Can you work these out from the model? Positions are in its coordinate system, mm. A direction names the side the tool comes from. Give positions to 0.01 mm unless a question says otherwise; leave off trailing zeros. Loops run counter-clockwise (first coordinate to the right, second up) from the corner with the lowest first, then second, coordinate; pieces in that order, holes last. Notation, with made-up numbers: (87.5, 87) -> (91.5, 87) arc R14 ccw to (91.5, 103) -> close; hole circle Ø8 at (-39, -35.75). An arc over 180 degrees is marked (long way). One line per question, with ' | ' between items.
from build123d import *

# Parameters (mm, degrees)
F0_R     = 85
F5_R     = 11
F6_DEPTH = 25
F7_R     = 142.5
F7_R_2   = 11
F7_R_3   = 85
F8_DEPTH = 25


with BuildPart() as f4:
    # F4: sweep along a path in F4_path
    with BuildLine(Plane(origin=(0, 0, 0), x_dir=(0, 1, 0), z_dir=(0, 0, 1))) as f4_path:
        Line((0, 0), (0, -30))
        ThreePointArc((0, -30), (-49.7918471983, -150.2081528017), (-170, -200))
        Line((-170, -200), (-1710, -200))
    # F0 (on Right) → F4 (sweep)
    with BuildSketch(Plane.YZ):
        Circle(F0_R)
    sweep(path=f4_path.line)

    # F5 (on face) → F6 (join)
    with BuildSketch(Plane.XZ.offset(1710)):
        with BuildLine():
            ThreePointArc((84.4, 10.0816665289), (78.6809157211, 32.1607447254), (67.296875, 51.9242777055))
            ThreePointArc((67.296875, 51.9242777055), (57.5, 0), (67.296875, -51.9242777055))
            ThreePointArc((67.296875, -51.9242777055), (78.6809157211, -32.1607447254), (84.4, -10.0816665289))
            ThreePointArc((84.4, -10.0816665289), (69, 0), (84.4, 10.0816665289))
        make_face()
        with BuildLine():
            ThreePointArc((67.296875, -51.9242777055), (226.4202071103, -140.0293635501), (342.5, 0))
            ThreePointArc((342.5, 0), (226.4202071103, 140.0293635501), (67.296875, 51.9242777055))
            ThreePointArc((67.296875, 51.9242777055), (78.6809157211, 32.1607447254), (84.4, 10.0816665289))
            ThreePointArc((84.4, 10.0816665289), (89.2032602919, 6.0249481326), (91, 0))
            ThreePointArc((91, 0), (89.2032602919, -6.0249481326), (84.4, -10.0816665289))
            ThreePointArc((84.4, -10.0816665289), (78.6809157211, -32.1607447254), (67.296875, -51.9242777055))
        make_face()
        with Locations((115.1471862576, -84.8528137424)):
            Circle(F5_R, mode=Mode.SUBTRACT)
        with Locations((200, -120)):
            Circle(F5_R, mode=Mode.SUBTRACT)
        with Locations((284.8528137424, -84.8528137424)):
            Circle(F5_R, mode=Mode.SUBTRACT)
        with Locations((115.1471862576, 84.8528137424)):
            Circle(F5_R, mode=Mode.SUBTRACT)
        with Locations((320, 0)):
            Circle(F5_R, mode=Mode.SUBTRACT)
        with Locations((200, 120)):
            Circle(F5_R, mode=Mode.SUBTRACT)
        with Locations((284.8528137424, 84.8528137424)):
            Circle(F5_R, mode=Mode.SUBTRACT)
    extrude(amount=-F6_DEPTH)

    # F7 (on face) → F8 (join)
    with BuildSketch(Plane(origin=(0, 0, 0), x_dir=(0, -1, 0), z_dir=(-1, 0, 0))):
        Circle(F7_R)
        with Locations((-82.4812086801, -82.4812086801)):
            Circle(F7_R_2, mode=Mode.SUBTRACT)
        with Locations((0, -116.6460439563)):
            Circle(F7_R_2, mode=Mode.SUBTRACT)
        with Locations((82.4812086801, -82.4812086801)):
            Circle(F7_R_2, mode=Mode.SUBTRACT)
        with Locations((-116.6460439563, 0)):
            Circle(F7_R_2, mode=Mode.SUBTRACT)
        with Locations((-82.4812086801, 82.4812086801)):
            Circle(F7_R_2, mode=Mode.SUBTRACT)
        Circle(F7_R_3, mode=Mode.SUBTRACT)
        with Locations((116.6460439563, 0)):
            Circle(F7_R_2, mode=Mode.SUBTRACT)
        with Locations((0, 116.6460439563)):
            Circle(F7_R_2, mode=Mode.SUBTRACT)
        with Locations((82.4812086801, 82.4812086801)):
            Circle(F7_R_2, mode=Mode.SUBTRACT)
    extrude(amount=-F8_DEPTH)


solid = f4.part
Q1. For pin 1 Ø20 at (y, z) = (-116.65, 0) entering from +X; pin 2 Ø10 at (y, z) = (-1335, 3.5) entering from -X; pin 3 Ø1 at (y, z) = (-580.5, -61) entering from -X; pin 4 Ø17.5 at (y, z) = (0, -116.65) entering from +X, each with a flat end and sliding along its axis, tell me the tip position at first contact or that it passes through.
Entries:
pin 1: x = 281.29 | pin 2: x = 115 | pin 3: x = 140.29 | pin 4: through
Q2. On a 3-axis mill with a long thin cutter (end or side, diameter ignored), from which of +Z, -Z, +X, -X, +Y, -Y can I reach the whole of each face in a straight line? I mean faces 1 (the face through (198, -1710, 2)), 2 (the face through (27.535, -67.453, -51.721)). Say none if no direction works.
Entries:
face 1: +Z, -Z, +X, -X, -Y | face 2: none
Q3. If we section it at A-A (y = -190): Write out the boundary of the cut face in (x, z).
Entries:
outline: circle Ø170 at (200, 0)
Q4. If I drill on probe 1 along Z at (x, y) = (17.5, 0); probe 2 along Y at (x, z) = (128, -57.5); probe 3 along Z at (x, y) = (175.5, -710), over which ranges is the centre line in solid material (lowest first)? Write a range as from..to.
Entries:
probe 1: -142.5..-127.65, -105.65..105.65, 127.65..142.5 | probe 2: -1710..-1685, -126.06..40.95 | probe 3: -81.39..81.39
Q5. If we mould it in two halves opening along Y, with no side actions, what happens to faces 3 (the face through (12.325, 105.028, 96.308)), 4 (the face through (0, 2, 2)), 5 (the face through (261, -1685, -61))? For each: pulls with the +Y half, pulls with the -Y half, needs draft (parallel to the pull), parting line crosses it, or undercut.
Entries:
face 3: parting line crosses it | face 4: needs draft | face 5: undercut
